from build123d import *

# Parameters (mm, degrees)
SKETCH1_W           = 30
SKETCH1_H           = 60
BOSS_EXTRUDE1_DEPTH = 5
SKETCH2_W           = 30
SKETCH2_H           = 5
BOSS_EXTRUDE2_DEPTH = 40
BOSS_EXTRUDE3_DEPTH = 7
FILLET1_R           = 2
SKETCH4_W           = 5
SKETCH4_H           = 60
BOSS_EXTRUDE4_DEPTH = 25
SKETCH5_W           = 5
SKETCH5_H           = 60
BOSS_EXTRUDE5_DEPTH = 25
FILLET2_R           = 8
SKETCH6_R           = 1.5
CUT_EXTRUDE1_DEPTH  = 5
FILLET3_R           = 8
CUT_EXTRUDE2_REACH  = 87
SKETCH7_W           = 18
SKETCH7_H           = 4
CUT_EXTRUDE4_DEPTH  = 2


with BuildPart() as part:
    # Sketch1 → Boss-Extrude1 (new body)
    with BuildSketch(Plane.XY):
        Rectangle(SKETCH1_W, SKETCH1_H)
    extrude(amount=-BOSS_EXTRUDE1_DEPTH)

    # Sketch2 → Boss-Extrude2 (add)
    with BuildSketch(Plane(origin=(0, 0, -5), x_dir=(-1, 0, 0), z_dir=(0, 0, -1))):
        with Locations((0, -27.5)):
            Rectangle(SKETCH2_W, SKETCH2_H)
        with Locations((0, 27.5)):
            Rectangle(SKETCH2_W, SKETCH2_H)
    extrude(amount=BOSS_EXTRUDE2_DEPTH)

    # Sketch3 → Boss-Extrude3 (add)
    with BuildSketch(Plane(origin=(0, 0, -5), x_dir=(-1, 0, 0), z_dir=(0, 0, -1))):
        with BuildLine():
            Line((4, -2.5), (-4, -2.5))
            ThreePointArc((-4, -2.5), (-5.414213562, -1.914213562), (-6, -0.5))
            Line((-6, -0.5), (-6, 0.5))
            ThreePointArc((-6, 0.5), (-5.414213562, 1.914213562), (-4, 2.5))
            Line((-4, 2.5), (4, 2.5))
            ThreePointArc((4, 2.5), (5.414213562, 1.914213562), (6, 0.5))
            Line((6, 0.5), (6, -0.5))
            ThreePointArc((6, -0.5), (5.414213562, -1.914213562), (4, -2.5))
        make_face()
    extrude(amount=BOSS_EXTRUDE3_DEPTH)

    # Fillet1
    fillet1_edges = [part.edges().sort_by_distance(p)[0] for p in [
        (0, -25, -5),
        (0, 25, -5),
    ]]
    fillet(fillet1_edges, radius=FILLET1_R)

    # Sketch4 → Boss-Extrude4 (add)
    with BuildSketch(Plane(origin=(15, 0, 0), x_dir=(0, 0, -1), z_dir=(1, 0, 0))):
        with Locations((2.5, 0)):
            Rectangle(SKETCH4_W, SKETCH4_H)
    extrude(amount=BOSS_EXTRUDE4_DEPTH)

    # Sketch5 → Boss-Extrude5 (add)
    with BuildSketch(Plane.ZY.offset(15)):
        with Locations((-2.5, 0)):
            Rectangle(SKETCH5_W, SKETCH5_H)
    extrude(amount=BOSS_EXTRUDE5_DEPTH)

    # Fillet2
    fillet2_edges = [part.edges().sort_by_distance(p)[0] for p in [
        (40, 30, -2.5),
        (40, -30, -2.5),
        (-40, -30, -2.5),
        (-40, 30, -2.5),
    ]]
    fillet(fillet2_edges, radius=FILLET2_R)

    # Sketch6 → Cut-Extrude1 (cut)
    with BuildSketch(Plane(origin=(0, 0, -5), x_dir=(-1, 0, 0), z_dir=(0, 0, -1))):
        with Locations((33, -23)):
            Circle(SKETCH6_R)
        with Locations(Location((-33, -23, 0), (0, 0, 180))):
            Circle(SKETCH6_R)
        with Locations((-33, 23)):
            Circle(SKETCH6_R)
        with Locations(Location((33, 23, 0), (0, 0, 180))):
            Circle(SKETCH6_R)
    extrude(amount=-CUT_EXTRUDE1_DEPTH, mode=Mode.SUBTRACT)

    # Fillet3
    fillet3_edges = [part.edges().sort_by_distance(p)[0] for p in [
        (-15, -27.5, -45),
        (15, -27.5, -45),
        (-15, 27.5, -45),
        (15, 27.5, -45),
    ]]
    fillet(fillet3_edges, radius=FILLET3_R)

    # Cut-Extrude2: up to this face of the body (flat: up to its plane)
    cut_extrude2_end = Plane(part.part.faces().sort_by_distance((0, -30, -19.840780346))[0])
    # Sketch7 → Cut-Extrude2 (cut, up to the picked face)
    with BuildSketch(Plane(origin=(0, 30, 0), x_dir=(1, 0, 0), z_dir=(0, 1, 0)), mode=Mode.PRIVATE) as cut_extrude2_sk1:
        with Locations((0, 36)):
            Rectangle(SKETCH7_W, SKETCH7_H)
    cut_extrude2_tool1 = split(extrude(cut_extrude2_sk1.sketch, amount=-CUT_EXTRUDE2_REACH, mode=Mode.PRIVATE), bisect_by=cut_extrude2_end, keep=Keep.BOTH, mode=Mode.PRIVATE)
    add(cut_extrude2_tool1.solids().sort_by(Axis((0, 30, -36), (0, -1, 0)))[0], mode=Mode.SUBTRACT)

    # Sketch10 → Cut-Extrude4 (cut)
    with BuildSketch(Plane.XY):
        with BuildLine():
            Line((32, 30), (-32, 30))
            ThreePointArc((-32, 30), (-37.656854249, 27.656854249), (-40, 22))
            Line((-40, 22), (-40, -22))
            ThreePointArc((-40, -22), (-37.656854249, -27.656854249), (-32, -30))
            Line((-32, -30), (32, -30))
            ThreePointArc((32, -30), (37.656854249, -27.656854249), (40, -22))
            Line((40, -22), (40, 22))
            ThreePointArc((40, 22), (37.656854249, 27.656854249), (32, 30))
        make_face()
    extrude(amount=-CUT_EXTRUDE4_DEPTH, mode=Mode.SUBTRACT)


solid = part.part
Read the model definition and answer for the solid it produces. Units are mm, in the model's axes. A direction names the side the tool comes from. Round coordinates to 2 decimals unless told otherwise and drop trailing zeros. Write each loop counter-clockwise with the first axis right and the second up, starting at its lowest first coordinate (ties: lowest second). Pieces come first, ordered by that corner, then holes. Notation, with made-up numbers: (42, 85.25) - (90, 85.25) arc R17 cw to (90, 117.25) - close; hole circle Ø2 at (82, 75.5). An arc over 180 degrees is marked (long way). Use a Markdown table: item, result.
(1) The part is cut by section B-B (z = -22.5). Write down the section's boundary in (x, y).
Reported:
| item | result |
|---|---|
| outline | (-15, -30) - (15, -30) - (15, -25) - (-15, -25) - close; (-15, 25) - (15, 25) - (15, 30) - (-15, 30) - close |
(2) Straight lines are drawn through the part: line 1 along Y through (x, z) = (12, -16.5); line 2 along Y through (x, z) = (-33, -3); line 3 along Z through (x, y) = (19, 13). For each, find the intervals that lie inside material, in ascending order. Write a range as [from, to].
Reported:
| item | result |
|---|---|
| line 1 | [-30, -25], [25, 30] |
| line 2 | [-29.94, -24.5], [-21.5, 21.5], [24.5, 29.94] |
| line 3 | [-5, -2] |
(3) The mould has two halves that part along X. Classify faces 4 (the cylindrical face through (31.89, -24.01, -3.52)), 5 (the flat face through (9, -27, -36)), 6 (the flat face through (-15, 27, -21)), 7 (the flat face through (40, 0, -3)): released by +X, released by -X, zero draft, split by the parting line, or undercut.
Reported:
| item | result |
|---|---|
| face 4 | undercut |
| face 5 | undercut |
| face 6 | released by -X |
| face 7 | released by +X |
(4) The part is cut by section A-A (x = -0.5). Write down the section's boundary in (y, z).
Reported:
| item | result |
|---|---|
| outline | (-30, -45) - (-25, -45) - (-25, -38) - (-30, -38) - close; (-30, -34) - (-25, -34) - (-25, -7) arc R2 cw to (-23, -5) - (-2.5, -5) - (-2.5, -12) - (2.5, -12) - (2.5, -5) - (23, -5) arc R2 cw to (25, -7) - (25, -34) - (30, -34) - (30, -2) - (-30, -2) - close; (25, -45) - (30, -45) - (30, -38) - (25, -38) - close |
(5) The part is cut by section D-D (y = 8.5). Write down the section's boundary in (x, z).
Reported:
| item | result |
|---|---|
| outline | (-40, -5) - (40, -5) - (40, -2) - (-40, -2) - close |
(6) Each of these flat-tipped pins is pushed along its axis until it touches: pin 1 Ø5 at (x, y) = (20.5, -21.5) entering from -Z; pin 2 Ø2 at (y, z) = (23, -20) entering from -X; pin 3 Ø0.8 at (y, z) = (0, -8) entering from -X; pin 4 Ø2 at (y, z) = (27.5, -35) entering from -X. Where does it stop, or does it pass through?
Reported:
| item | result |
|---|---|
| pin 1 | z = -5 |
| pin 2 | through |
| pin 3 | x = -6 |
| pin 4 | x = -15 |
(7) The part is cut by section C-C (x = 14). Write down the section's boundary in (y, z), then the cut area to 3 significant figures.
Reported:
| item | result |
|---|---|
| outline | (-30, -40.87) - (-25, -40.87) - (-25, -7) arc R2 cw to (-23, -5) - (23, -5) arc R2 cw to (25, -7) - (25, -40.87) - (30, -40.87) - (30, -2) - (-30, -2) - close |
| area | 540 mm2 |
(8) Which of the six approach directions +Z, -Z, +X, -X, +Y, -Y give full straight-line access (tool end or side, diameter ignored) to faces 1 (the cylindrical face through (5.43, 1.9, -8.45)), 2 (the flat face through (9, 28, -36)), 3 (the flat face through (0, 0, -12))?
Reported:
| item | result |
|---|---|
| face 1 | -Z, +X |
| face 2 | +Y, -Y |
| face 3 | -Z, +X, -X |
